Build history of the part. All positions in model axes, mm. A direction names the side the tool comes from. Give positions to 0.01 mm unless a question says otherwise; leave off trailing zeros. Order: outer loops, then holes, each group sorted by start corner. A loop starts at its lowest first (then second) coordinate and runs counter-clockwise, first axis right, second up. Notation, with made-up numbers: (-7.75, -5) -> (43.25, -5) arc R25 ccw to (43.25, 12) -> close; hole circle Ø2 at (67.5, 30). An arc over 180 degrees is marked (long way). One line per question, with ' | ' between items. Start each with the question number.
(1) Cut at C-C (y = -13.1). Give the cut face in (x, z), then the cut area to 3 significant figures.
(2) Cut at A-A (z = -1). Give the cut face in (x, y), then the cut area to 3 significant figures.
(3) Which spindle directions (+Z, -Z, +X, -X, +Y, -Y) get a long thin tool onto all of the face, cutting with end or side? Do faces 1 (the face through (0, 17, -1)), 2 (the face through (-2, 16, 4)), 3 (the face through (0.2, 7, 5)), 4 (the face through (-11.45, -13.04, -1.23)), 5 (the face through (-2, 11, 10.15)). Say none if no direction does.
(4) Drill centre lines: L1, parallel to Y at x = 10, z = -1.5; L2, parallel to Z at x = -4.75, y = 6.5; L3, parallel to X at y = 14, z = -0.5. Where is each one in solid material? Low to high. Write a range as from..to.
(5) Cut at B-B (x = 10). Give the cut face in (y, z), then the cut area to 3 significant figures.
(6) Cut at D-D (z = 6.25). Give the cut face in (x, y).
(7) Pin check, flat tips, straight feed: pin 1 Ø3.5 at (x, y) = (-10, 13.1) entering from +Z; pin 2 Ø1.5 at (x, z) = (0, 10.5) entering from +Y; pin 3 Ø1.2 at (x, z) = (-2.5, 5.5) entering from +Y; pin 4 Ø1.7 at (x, y) = (-10, -13.1) entering from -Z. Stop position of each tip, or through.
(8) Pull direction X, two halves, no side cores. Call faces 6 (the face through (13.1, 0, -1)), 7 (the face through (8.55, -13.04, -1.23)), 8 (the face through (-1.77, -7.07, 1.89)): +X half, -X half, draft (parallel to the pull), parting line (faces both ways), or undercut.
from build123d import *

# Parameters (mm, degrees)
SKETCH_R     = 1.45
PAD_DEPTH    = 2.5
PAD001_DEPTH = 2


with BuildPart() as part:
    # Sketch → Pad (new body)
    with BuildSketch(Plane.XY):
        with BuildLine():
            ThreePointArc((-12.1, 17), (-12.807107, 16.707107), (-13.1, 16))
            Line((-13.1, -16), (-13.1, 16))
            ThreePointArc((-13.1, -16), (-12.807107, -16.707107), (-12.1, -17))
            Line((12.1, -17), (-12.1, -17))
            ThreePointArc((12.1, -17), (12.807107, -16.707107), (13.1, -16))
            Line((13.1, 16), (13.1, -16))
            ThreePointArc((13.1, 16), (12.807107, 16.707107), (12.1, 17))
            Line((-12.1, 17), (12.1, 17))
        make_face()
        with Locations((10, 13.1)):
            Circle(SKETCH_R, mode=Mode.SUBTRACT)
        with Locations((-10, 13.1)):
            Circle(SKETCH_R, mode=Mode.SUBTRACT)
        with Locations((-10, -13.1)):
            Circle(SKETCH_R, mode=Mode.SUBTRACT)
        with Locations((10, -13.1)):
            Circle(SKETCH_R, mode=Mode.SUBTRACT)
    extrude(amount=-PAD_DEPTH)

    # Sketch001 → Pad001 (join, symmetric)
    with BuildSketch(Plane.YZ.offset(-1.8)):
        with BuildLine():
            ThreePointArc((16, 8), (12.294095, 12.829629), (6.669873, 10.5))
            Line((6.669873, 10.5), (3.585892, 5.158388))
            ThreePointArc((1.60844, 3.723286), (2.749885, 4.230403), (3.585892, 5.158388))
            Line((1.60844, 3.723286), (-16, 0))
            Line((-16, 0), (16, 0))
            Line((16, 8), (16, 0))
        make_face()
        with BuildLine():
            Line((9.47972, 9.52028), (10.109441, 10.15))
            Line((10.109441, 10.15), (11.890559, 10.15))
            Line((11.890559, 10.15), (12.52028, 9.52028))
            ThreePointArc((9.47972, 9.52028), (11, 5.85), (12.52028, 9.52028))
        make_face(mode=Mode.SUBTRACT)
    extrude(amount=PAD001_DEPTH, both=True)


solid = part.part
Result set:
1) outline: (-13.1, -2.5) -> (-11.45, -2.5) -> (-11.45, 0) -> (-13.1, 0) -> close; (-8.55, -2.5) -> (8.55, -2.5) -> (8.55, 0) -> (0.2, 0) -> (0.2, 0.61) -> (-3.8, 0.61) -> (-3.8, 0) -> (-8.55, 0) -> close; (11.45, -2.5) -> (13.1, -2.5) -> (13.1, 0) -> (11.45, 0) -> close | area: 53.5 mm2
2) outline: (-13.1, -16) arc R1 ccw to (-12.1, -17) -> (12.1, -17) arc R1 ccw to (13.1, -16) -> (13.1, 16) arc R1 ccw to (12.1, 17) -> (-12.1, 17) arc R1 ccw to (-13.1, 16) -> close; hole circle Ø2.9 at (-10, -13.1); hole circle Ø2.9 at (-10, 13.1); hole circle Ø2.9 at (10, -13.1); hole circle Ø2.9 at (10, 13.1) | area: 864 mm2
3) face 1: +Z, -Z, +X, -X, +Y | face 2: +Z, +X, -X, +Y | face 3: +Z, +X, +Y, -Y | face 4: +Z, -Z | face 5: +X, -X
4) L1: y = -17..-14.55, -11.65..11.65, 14.55..17 | L2: z = -2.5..0 | L3: x = -13.1..-11.14, -8.86..8.86, 11.14..13.1
5) outline: (-17, -2.5) -> (-14.55, -2.5) -> (-14.55, 0) -> (-17, 0) -> close; (-11.65, -2.5) -> (11.65, -2.5) -> (11.65, 0) -> (-11.65, 0) -> close; (14.55, -2.5) -> (17, -2.5) -> (17, 0) -> (14.55, 0) -> close | area: 70.5 mm2
6) outline: (-3.8, 4.22) -> (0.2, 4.22) -> (0.2, 9.75) -> (-3.8, 9.75) -> close; (-3.8, 12.25) -> (0.2, 12.25) -> (0.2, 16) -> (-3.8, 16) -> close
7) pin 1: stops at z = 0 | pin 2: stops at y = 15.68 | pin 3: stops at y = 16 | pin 4: passes through
8) face 6: +X half | face 7: undercut | face 8: draft
